from build123d import *

# Parameters (mm, degrees)
SKETCH1_R           = 14
BOSS_EXTRUDE1_DEPTH = 3
CUT_EXTRUDE1_DEPTH  = 4
FILLET1_R           = 1


with BuildPart() as part:
    # Sketch1 → Boss-Extrude1 (new body)
    with BuildSketch(Plane(origin=(0, 0, 0), x_dir=(1, 0, 0), z_dir=(0, 1, 0))):
        with BuildLine():
            Line((3.491378029, 30.5), (-3.491378029, 30.5))
            ThreePointArc((-3.491378029, 30.5), (-5.40479519, 30.119397663), (-7.026911935, 29.035533906))
            Line((-7.026911935, 29.035533906), (-29.035533906, 7.026911935))
            ThreePointArc((-29.035533906, 7.026911935), (-30.119397663, 5.40479519), (-30.5, 3.491378029))
            Line((-30.5, 3.491378029), (-30.5, -3.491378029))
            ThreePointArc((-30.5, -3.491378029), (-30.119397663, -5.40479519), (-29.035533906, -7.026911935))
            Line((-29.035533906, -7.026911935), (-7.026911935, -29.035533906))
            ThreePointArc((-7.026911935, -29.035533906), (-5.40479519, -30.119397663), (-3.491378029, -30.5))
            Line((-3.491378029, -30.5), (3.491378029, -30.5))
            ThreePointArc((3.491378029, -30.5), (5.40479519, -30.119397663), (7.026911935, -29.035533906))
            Line((7.026911935, -29.035533906), (29.035533906, -7.026911935))
            Line((29.035533906, -7.026911935), (27.5, -3.491378029))
            Line((27.5, -3.491378029), (27.5, 3.491378029))
            Line((27.5, 3.491378029), (29.035533906, 7.026911935))
            Line((29.035533906, 7.026911935), (7.026911935, 29.035533906))
            ThreePointArc((7.026911935, 29.035533906), (5.40479519, 30.119397663), (3.491378029, 30.5))
        make_face()
        Circle(SKETCH1_R, mode=Mode.SUBTRACT)
    extrude(amount=BOSS_EXTRUDE1_DEPTH)

    # Sketch2 → Cut-Extrude1 (cut, through all)
    with BuildSketch(Plane(origin=(0, 3, 0), x_dir=(1, 0, 0), z_dir=(0, 1, 0))):
        Polygon((-26.25, 7.929437252), (-26.25, 6.129437252), (-24.9, 6.129437252), (-24.9, 4.779437252), (-23.1, 4.779437252), (-23.1, 6.129437252), (-21.75, 6.129437252), (-21.75, 7.929437252), (-23.1, 7.929437252), (-23.1, 9.279437252), (-24.9, 9.279437252), (-24.9, 7.929437252), align=None)
        Polygon((-23.1, -4.779437252), (-24.9, -4.779437252), (-24.9, -6.129437252), (-26.25, -6.129437252), (-26.25, -7.929437252), (-24.9, -7.929437252), (-24.9, -9.279437252), (-23.1, -9.279437252), (-23.1, -7.929437252), (-21.75, -7.929437252), (-21.75, -6.129437252), (-23.1, -6.129437252), align=None)
        Polygon((7.929437252, 23.1), (9.279437252, 23.1), (9.279437252, 24.9), (7.929437252, 24.9), (7.929437252, 26.25), (6.129437252, 26.25), (6.129437252, 24.9), (4.779437252, 24.9), (4.779437252, 23.1), (6.129437252, 23.1), (6.129437252, 21.75), (7.929437252, 21.75), align=None)
        Polygon((26.25, -7.929437252), (26.25, -6.129437252), (24.9, -6.129437252), (24.9, -4.779437252), (23.1, -4.779437252), (23.1, -6.129437252), (21.75, -6.129437252), (21.75, -7.929437252), (23.1, -7.929437252), (23.1, -9.279437252), (24.9, -9.279437252), (24.9, -7.929437252), align=None)
        Polygon((-4.779437252, 24.9), (-6.129437252, 24.9), (-6.129437252, 26.25), (-7.929437252, 26.25), (-7.929437252, 24.9), (-9.279437252, 24.9), (-9.279437252, 23.1), (-7.929437252, 23.1), (-7.929437252, 21.75), (-6.129437252, 21.75), (-6.129437252, 23.1), (-4.779437252, 23.1), align=None)
        Polygon((26.25, 7.929437252), (24.9, 7.929437252), (24.9, 9.279437252), (23.1, 9.279437252), (23.1, 7.929437252), (21.75, 7.929437252), (21.75, 6.129437252), (23.1, 6.129437252), (23.1, 4.779437252), (24.9, 4.779437252), (24.9, 6.129437252), (26.25, 6.129437252), align=None)
        Polygon((-6.129437252, -26.25), (-6.129437252, -24.9), (-4.779437252, -24.9), (-4.779437252, -23.1), (-6.129437252, -23.1), (-6.129437252, -21.75), (-7.929437252, -21.75), (-7.929437252, -23.1), (-9.279437252, -23.1), (-9.279437252, -24.9), (-7.929437252, -24.9), (-7.929437252, -26.25), align=None)
        Polygon((7.929437252, -26.25), (7.929437252, -24.9), (9.279437252, -24.9), (9.279437252, -23.1), (7.929437252, -23.1), (7.929437252, -21.75), (6.129437252, -21.75), (6.129437252, -23.1), (4.779437252, -23.1), (4.779437252, -24.9), (6.129437252, -24.9), (6.129437252, -26.25), align=None)
    extrude(amount=-CUT_EXTRUDE1_DEPTH, mode=Mode.SUBTRACT)

    # Fillet1
    fillet1_edges = [part.edges().sort_by_distance(p)[0] for p in [
        (29.035533906, 1.5, -7.026911935),
        (27.5, 1.5, -3.491378029),
        (27.5, 1.5, 3.491378029),
        (29.035533906, 1.5, 7.026911935),
    ]]
    fillet(fillet1_edges, radius=FILLET1_R)


solid = part.part
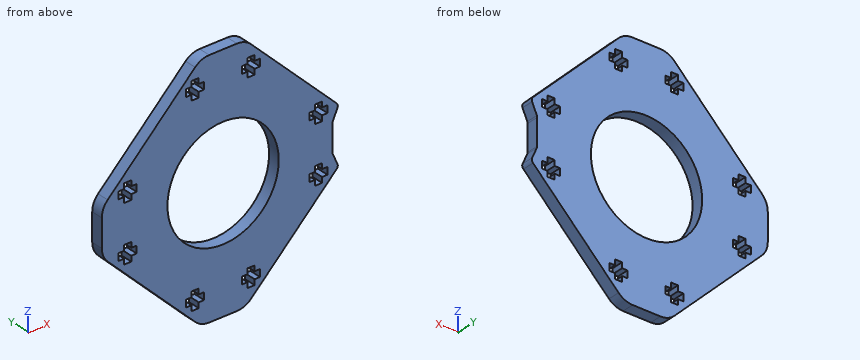
Verification items for the finished model (mm, model axes). Round coordinates to 2 decimals unless told otherwise and drop trailing zeros. Order: outer loops, then holes, each group sorted by start corner. A loop starts at its lowest first (then second) coordinate and runs counter-clockwise, first axis right, second up. Notation, with made-up numbers: (9, -36) -> (38, -36) arc R33 cw to (38, -4) -> close; hole circle Ø7 at (17.5, -10.75). An arc over 180 degrees is marked (long way). Put each result on its own line as item: value.
1) Depth check by flat-ended pin: pin 1 (0.7 mm diameter, centred on y = 1, z = -5, fed in from +X); pin 2 (0.9 mm diameter, centred on y = 1.5, z = -23.5, fed in from -X); pin 3 (0.5 mm diameter, centred on y = 1.5, z = 24, fed in from +X). Enter the tip coordinate at first touch or a pass-through.
Final values:
pin 1: stops at x = 28.31
pin 2: stops at x = -13.01
pin 3: stops at x = 12.31
2) Material ranges on line 1 (Z direction, x = 0, y = 1); line 2 (X direction, y = 1.1, z = 0); line 3 (X direction, y = 2.05, z = -9), recorded low to high.
Final values:
line 1: z = -30.5 to -14, 14 to 30.5
line 2: x = -30.5 to -14, 14 to 27.5
line 3: x = -27.06 to -24.9, -23.1 to -10.72, 10.72 to 23.1, 24.9 to 27.06
3) Section check D-D (y = 1.4). Give the number of separate pieces and of enclosed holes in the cut face, then the cut area to 3 significant figures.
Final values:
separate pieces: 1
enclosed holes: 9
area: 1,720 mm^2
4) Section check A-A (z = 0). Record the cut outline in (x, y).
Final values:
outline: (-30.5, 0) -> (-14, 0) -> (-14, 3) -> (-30.5, 3) -> close; (14, 0) -> (27.5, 0) -> (27.5, 3) -> (14, 3) -> close
5) Section check C-C (z = 24). Record the cut outline in (x, y).
Final values:
outline: (-12.06, 0) -> (-9.28, 0) -> (-9.28, 3) -> (-12.06, 3) -> close; (-4.78, 0) -> (4.78, 0) -> (4.78, 3) -> (-4.78, 3) -> close; (9.28, 0) -> (12.06, 0) -> (12.06, 3) -> (9.28, 3) -> close
6) Section check B-B (x = 0). Record the cut outline in (y, z).
Final values:
outline: (0, -30.5) -> (3, -30.5) -> (3, -14) -> (0, -14) -> close; (0, 14) -> (3, 14) -> (3, 30.5) -> (0, 30.5) -> close
